from build123d import *

# Parameters (mm, degrees)
ESQUISSE1_W                           = 100
ESQUISSE1_H                           = 100
BOSS_EXTRU_1_DEPTH                    = 80
ESQUISSE2_W                           = 86
ESQUISSE2_H                           = 86
ENL_V_MAT_EXTRU_1_DEPTH               = 70
ESQUISSE4_R                           = 9.5
ESQUISSE4_R_2                         = 1.5
BOSS_EXTRU_3_DEPTH                    = 3
CONG_1_R                              = 7
CONG_4_R                              = 9.5
D_GAGEMENT_M31_D                      = 3.4
D_GAGEMENT_M31_DEPTH                  = 3
ENL_V_MAT_EXTRU_2_REACH               = 184.154
ENL_V_MAT_EXTRU_2_OFFSET_FROM_SURFACE = 7
ESQUISSE8_W                           = 86
ESQUISSE8_H                           = 15
ENL_V_START                           = -13.296333
ENL_V_MAT_EXTRU_3_DEPTH               = 112.592666


with BuildPart() as part:
    # Esquisse1 → Boss.-Extru.1 (new body)
    with BuildSketch(Plane.XY):
        with Locations((50, 50)):
            Rectangle(ESQUISSE1_W, ESQUISSE1_H)
    extrude(amount=BOSS_EXTRU_1_DEPTH)

    # Esquisse2 → Enlèv. mat.-Extru.1 (cut)
    with BuildSketch(Plane(origin=(0, 0, 0), x_dir=(-1, 0, 0), z_dir=(0, 0, -1))):
        with Locations((-50, 50)):
            Rectangle(ESQUISSE2_W, ESQUISSE2_H)
    extrude(amount=-ENL_V_MAT_EXTRU_1_DEPTH, mode=Mode.SUBTRACT)

    # Esquisse4 → Boss.-Extru.3 (add)
    # profile 1 of 3: a face of its own
    with BuildSketch(Plane(origin=(0, 0, 0), x_dir=(-1, 0, 0), z_dir=(0, 0, -1))):
        with Locations((0.610912703, -0.610912703)):
            Circle(ESQUISSE4_R)
        with Locations((4.5, -4.5)):
            Circle(ESQUISSE4_R_2, mode=Mode.SUBTRACT)
    # profile 2 of 3: a face of its own
    with BuildSketch(Plane(origin=(0, 0, 0), x_dir=(-1, 0, 0), z_dir=(0, 0, -1))):
        with Locations((-100.610912703, -0.610912703)):
            Circle(ESQUISSE4_R)
        with Locations((-104.5, -4.5)):
            Circle(ESQUISSE4_R_2, mode=Mode.SUBTRACT)
    # profile 3 of 3: a face of its own
    with BuildSketch(Plane(origin=(0, 0, 0), x_dir=(-1, 0, 0), z_dir=(0, 0, -1))):
        with BuildLine():
            Line((-46.958618735, 93), (-53.041381265, 93))
            ThreePointArc((-53.041381265, 93), (-50, 111.5), (-46.958618735, 93))
        make_face()
        with Locations((-50, 107.5)):
            Circle(ESQUISSE4_R_2, mode=Mode.SUBTRACT)
    extrude(amount=-BOSS_EXTRU_3_DEPTH)

    # Congé1
    cong_1_edges = [part.edges().sort_by_distance(p)[0] for p in [
        (0, 100, 40),
        (100, 100, 40),
        (100, 0, 41.5),
        (0, 0, 41.5),
    ]]
    fillet(cong_1_edges, radius=CONG_1_R)

    # Congé4
    cong_4_edges = [part.edges().sort_by_distance(p)[0] for p in [
        (91.130575913, 0, 1.5),
        (100, 8.869424087, 1.5),
        (0, 8.869424087, 1.5),
        (8.869424087, 0, 1.5),
        (40.712912189, 100, 1.5),
        (59.287087811, 100, 1.5),
    ]]
    fillet(cong_4_edges, radius=CONG_4_R)

    # Dégagement M31
    with Locations(Plane.XY.offset(3)):
        with Locations((104.5, -4.5), (-4.5, -4.5), (50, 107.5)):
            Hole(D_GAGEMENT_M31_D / 2, depth=D_GAGEMENT_M31_DEPTH)

    # Enlèv. mat.-Extru.2: up to this face of the body (flat: up to its plane, moved by the offset)
    enl_v_mat_extru_2_end = Plane(part.part.faces().sort_by_distance((50, 0, 40.310761501))[0]).offset(ENL_V_MAT_EXTRU_2_OFFSET_FROM_SURFACE)
    # Esquisse8 → Enlèv. mat.-Extru.2 (cut, up to the picked face)
    with BuildSketch(Plane(origin=(0, 102.060853814, 2.721755672), x_dir=(1, 0, 0), z_dir=(0, 0.9996445992724862, 0.026658491055395153)), mode=Mode.PRIVATE) as enl_v_mat_extru_2_sk1:
        with Locations((50, -8.834150894)):
            Rectangle(ESQUISSE8_W, ESQUISSE8_H)
    enl_v_mat_extru_2_tool1 = split(extrude(enl_v_mat_extru_2_sk1.sketch, amount=-ENL_V_MAT_EXTRU_2_REACH, mode=Mode.PRIVATE), bisect_by=enl_v_mat_extru_2_end, keep=Keep.BOTH, mode=Mode.PRIVATE)
    add(enl_v_mat_extru_2_tool1.solids().sort_by(Axis((50, 101.825349, 11.552767), (0, -0.9996445992724862, -0.026658491055395153)))[0], mode=Mode.SUBTRACT)

    # Esquisse9 → Enlèv. mat.-Extru.3 (cut)
    with BuildSketch(Plane.ZY.offset(-93).offset(ENL_V_START)):
        Polygon((18.820079232, 93), (16.52663391, 7), (1.521301003, 7), (3.814746326, 93), align=None)
    extrude(amount=ENL_V_MAT_EXTRU_3_DEPTH, mode=Mode.SUBTRACT)


solid = part.part
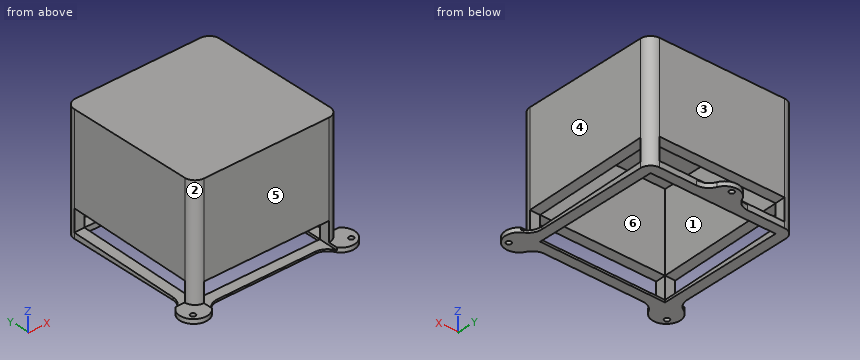
Input: part model. Units: mm. Frame: model coordinates. Face numbers are marked on the shaded views. A direction names the side the tool comes from. Coordinates: 2 decimals unless noted, no trailing zeros. Loops run counter-clockwise (first coordinate to the right, second up) from the corner with the lowest first, then second, coordinate; pieces in that order, holes last. Notation, with made-up numbers: (-38.5, 16.25) - (-20.5, 16.25) arc R25 cw to (-20.5, 46.25) - close; hole circle Ø10 at (82, -22). An arc over 180 degrees is marked (long way). Answer in a Markdown table with one row per item. Add a question column.
Item 1: Line query: line 1 along Y through (x, z) = (40.5, 28.5); line 2 along Z through (x, y) = (22.5, 10). Output: solid intervals per line, ascending. Write a range as [from, to].
Item 2: Mould query, pull axis Y, two halves, no side actions, for the marked faces 4, 5 and 6. Classes: released by +Y, released by -Y, zero draft, split by the parting line, or undercut.
Item 3: Section query A-A on x = 50. Return the cut outline in (y, z), then the cut area to 3 significant figures.
Item 4: Contact query for flat-ended pins moving along their axis: P1, Ø16, axis at x = 38.5, z = 37, coming from the +Y side; P2, Ø3, axis at x = 104.5, y = -4.5, coming from the +Z side; P3, Ø6, axis at x = 65, y = 75.5, coming from the -Z side; P4, Ø5.5, axis at x = 5, z = 12, coming from the -Y side. Output: stop coordinate, or through.
Item 5: Section query C-C on z = 35. Return the cut outline in (x, y).
Item 6: Access query for the marked faces 1, 2 and 3. Directions: +Z, -Z, +X, -X, +Y, -Y. A direction counts if a zero-diameter tool reaches every point of the face in a straight line with its end or side. Return the directions, or none.
Item 7: Section query D-D on y = 4. Return the cut outline in (x, z), then the cut area to 3 significant figures.
Item 8: Section query B-B on x = 73. Return the cut outline in (y, z), then the cut area to 3 significant figures.
Recorded:
| question | item | result |
|---|---|---|
| 1 | line 1 | [0, 7], [93, 100] |
| 1 | line 2 | [70, 80] |
| 2 | face 4 | zero draft |
| 2 | face 5 | released by -Y |
| 2 | face 6 | undercut |
| 3 | outline | (0, 0) - (7, 0) - (7, 1.52) - (0, 1.33) - close; (0, 16.34) - (7, 16.53) - (7, 70) - (93, 70) - (93, 18.82) - (100, 19.01) - (100, 80) - (0, 80) - close; (93, 0) - (105.8, 0) - (105.8, 3) - (100, 3) - (100, 4) - (93, 3.81) - close; (109.2, 0) - (111.5, 0) - (111.5, 3) - (109.2, 3) - close |
| 3 | area | 1,790 mm^2 |
| 4 | P1 | y = 100 |
| 4 | P2 | through |
| 4 | P3 | z = 70 |
| 4 | P4 | y = 0 |
| 5 | outline | (0, 7) arc R7 ccw to (7, 0) - (93, 0) arc R7 ccw to (100, 7) - (100, 93) arc R7 ccw to (93, 100) - (7, 100) arc R7 ccw to (0, 93) - close; hole (7, 7) - (93, 7) - (93, 93) - (7, 93) - close |
| 6 | face 1 | -Z |
| 6 | face 2 | +Z, -X, -Y |
| 6 | face 3 | +Z, +X, -X, +Y |
| 7 | outline | (-8.92, 0) - (108.92, 0) - (108.92, 3) - (99.32, 3) - (99.32, 80) - (0.68, 80) - (0.68, 3) - (-8.92, 3) - close; hole (7, 1.44) - (93, 1.44) - (93, 16.45) - (7, 16.45) - close |
| 7 | area | 6,660 mm^2 |
| 8 | outline | (0, 0) - (7, 0) - (7, 1.52) - (0, 1.33) - close; (0, 16.34) - (7, 16.53) - (7, 70) - (93, 70) - (93, 18.82) - (100, 19.01) - (100, 80) - (0, 80) - close; (93, 0) - (100, 0) - (100, 4) - (93, 3.81) - close |
| 8 | area | 1,770 mm^2 |
